Autodesk Inventor part; units mm, degrees
ref_plane "Work Plane10" through (0, 5.1, -62.2) normal (0, 0, -1) x (0, 1, 0)
ref_plane "YZ Plane" through (0, 0, 0) normal (1, 0, 0) x (0, 1, 0)
ref_plane "XZ Plane" through (0, 0, 0) normal (0, 1, 0) x (-1, 0, 0)
sketch "Sketch1" plane through (0, 0, 0) normal (0, 0, 1) x (1, 0, 0)
  line L0 (0, 5.1) -> (0, 10.2)
  line L1 (38.3, 5.1) -> (38.3, 10.2)
  line L2 (0, 0) -> (0, 5.1)
  line L3 (38.3, 0) -> (38.3, 5.1)
  line L4 (40.3, -1) -> (40.3, 11.2)
  line L5 (40.3, -1) -> (40.3, -2)
  line L6 (40.3, -2) -> (-1, -2)
  line L7 (-1, -2) -> (-2, -2)
  line L8 (-2, -2) -> (-2, 11.2)
  line L9 (38.3, 5.1) -> (38.3, 10.4)
  line L10 (38.3, 10.4) -> (0, 10.4)
  line L11 (0, 10.4) -> (0, 5.1)
  line L12 (0, 12.4) -> (-2, 12.4)
  line L13 (-2, 12.4) -> (-2, 11.2)
  line L14 (0, 12.4) -> (40.3, 12.4)
  line L15 (40.3, 12.4) -> (40.3, 11.2)
  line L16 (38.3, 0) -> (38.3, -2)
  line L17 (0, 0) -> (0, -2)
  dimension "d108" = 5.3
extrude "Extrusion1" add sketch "Sketch1" against normal blind 12 contours L2 L17 L6 L7 L8 L13 L12 L14 L15 L4 L5 L16 L3 L1 L9 L10 L11 L0
sketch "Sketch2" plane through (0, 0, 0) normal (0, 0, 1) x (1, 0, 0)
  line L0 (3.5908, 8.23) -> (9.5908, 8.23)
  line L1 (9.5908, 8.23) -> (9.5908, 0)
  line L2 (3.5908, 0) -> (9.5908, 0)
  line L3 (3.5908, 8.23) -> (3.5908, 0)
  line L4 (40.3, 12.4) -> (-2, 12.4)
  line L5 (-2, 12.4) -> (-2, -2)
  line L6 (-2, -2) -> (15, -2)
  line L7 (15, -2) -> (40.3, -2)
  line L8 (38.3, -2) -> (40.3, -2)
  line L9 (40.3, -2) -> (40.3, 12.4)
  line L10 (40.3, -2) -> (40.3, 12.4)
  point P0 (39.3, 11.2)
  point P1 (15, 12.4)
  dimension "d4" = 6
ref_plane "Work Plane10" through (0, 5.1, -62.2) normal (0, 0, -1) x (0, 1, 0)
sketch "Sketch20" plane through (0, -2, -12) normal (1, 0, 0) x (0, 0, -1)
  line L0 (0, 14.4) -> (0, 0)
  line L1 (0, 2) -> (0, 0)
  line L2 (0, 0) -> (-12, 0)
  line L3 (-12, 0) -> (0, 0)
  line L4 (-12, 0) -> (-12, 2)
  line L5 (-12, 2) -> (0, 2)
extrude "Extrusion25" add sketch "Sketch20" along normal blind 1
sketch "Sketch21" plane through (38.3, -2, 0) normal (-1, 0, 0) x (0, 0, 1)
  line L0 (0, 2) -> (0, 0)
  line L1 (-12, 0) -> (-12, 2)
  line L2 (-12, 14.4) -> (-12, 0)
  line L3 (0, 2) -> (0, 0)
  line L4 (-12, 2) -> (0, 2)
  line L5 (0, 2) -> (2.5, 2)
  line L6 (0, 2) -> (0, 0)
  line L7 (0, 0) -> (-12, 0)
  line L8 (0, 0) -> (-12, 0)
extrude "Extrusion26" add sketch "Sketch21" along normal blind 1
extrude "Extrusion27" add sketch "Sketch2" along normal blind 6
properties part number "frame2"
CAD build for the part. Positions are in the model's coordinates, mm. A direction names the side the tool comes from. Round coordinates to 2 decimals unless told otherwise and drop trailing zeros. Write each loop counter-clockwise with the first axis right and the second up, starting at its lowest first coordinate (ties: lowest second). Pieces come first, ordered by that corner, then holes. Notation, with made-up numbers: M 15.5,3.25 L 34.5,3.25 A24 ccw 34.5,14.25 Z; hole C 62,57.5 d1. An arc over 180 degrees is marked long. Use a Markdown table: item, result. Add a question column.
1. Flat gauge pin, fed straight in: P1, Ø6, axis at x = 25.5, y = 4.5, coming from the -Z side. Where does the tip first touch, or does it go through?
2. Slice it at A-A on x = 8. Give the cut face in (y, z).
3. Slice it at C-C on y = 0.5. Give the cut face in (x, z).
4. Slice it at D-D on z = -5.5. Give the cut face in (x, y), then the cut area to 3 significant figures.
5. Pull direction X, two halves, no side cores. Call faces 6 (the face through (19, 5, 6)), 7 (the face through (40.3, 5, -3)), 8 (the face through (9.591, 4, 3)): released by +X, released by -X, zero draft, split by the parting line, or undercut.
6. Drill centre lines: probe 1 along X at (y, z) = (8, 0.25); probe 2 along X at (y, z) = (-0.5, -2.5); probe 3 along Z at (x, y) = (3, 9.25). Where is each one in solid material? Low to high.
7. Slice it at B-B on z = 2.25. Give the cut face in (x, y), then the cut area to 3 significant figures.
8. 3-axis set-ups, long thin cutter, end or side, ignore diameter. For faces 1 (the face through (0.5, 0, -5.9)), 2 (the face through (-2, 5, -3)), 3 (the face through (3.591, 4, 3)), 4 (the face through (1, -1, -6)), 5 (the face through (19, 11, -12)): which of +Z, -Z, +X, -X, +Y, -Y reach the whole face in a straight line?
Reply:
| question | item | result |
|---|---|---|
| 1 | P1 | stops at z = 0 |
| 2 | outline | M -2,0 L 0,0 L 0,6 L -2,6 Z; M 8.23,0 L 10.4,0 L 10.4,-12 L 12.4,-12 L 12.4,6 L 8.23,6 Z |
| 3 | outline | M -2,-12 L 0,-12 L 0,0 L 3.59,0 L 3.59,6 L -2,6 Z; M 9.59,0 L 38.3,0 L 38.3,-12 L 40.3,-12 L 40.3,6 L 9.59,6 Z |
| 4 | outline | M -2,-2 L 1,-2 L 1,0 L 0,0 L 0,10.4 L 38.3,10.4 L 38.3,0 L 37.3,0 L 37.3,-2 L 40.3,-2 L 40.3,12.4 L -2,12.4 Z |
| 4 | area | 138 mm^2 |
| 5 | face 6 | zero draft |
| 5 | face 7 | released by +X |
| 5 | face 8 | undercut |
| 6 | probe 1 | x = -2 to 3.59, 9.59 to 40.3 |
| 6 | probe 2 | x = -2 to 1, 37.3 to 40.3 |
| 6 | probe 3 | z = 0 to 6 |
| 7 | outline | M -2,-2 L 40.3,-2 L 40.3,12.4 L -2,12.4 Z; hole M 3.59,0 L 9.59,0 L 9.59,8.23 L 3.59,8.23 Z |
| 7 | area | 560 mm^2 |
| 8 | face 1 | -Z |
| 8 | face 2 | +Z, -Z, -X, +Y, -Y |
| 8 | face 3 | +Z, -Z |
| 8 | face 4 | -Z, -Y |
| 8 | face 5 | -Z, +X, -X, +Y, -Y |
